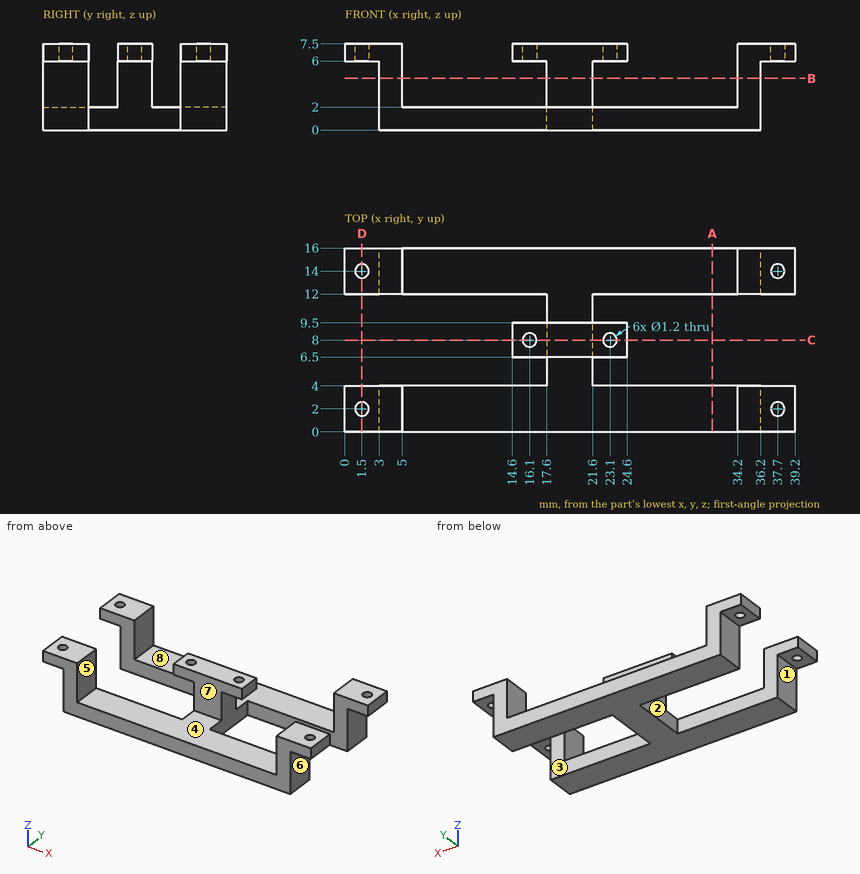
Input: dimensioned drawing with shaded views. Units: mm. Origin: part minimum x, y, z. A direction names the side the tool comes from. Give positions to 0.01 mm unless a question says otherwise; leave off trailing zeros. Order: outer loops, then holes, each group sorted by start corner. A loop starts at its lowest first (then second) coordinate and runs counter-clockwise, first axis right, second up. Notation, with made-up numbers: (28, -37) -> (40, -37) arc R12 cw to (40, -24) -> close; hole circle Ø3 at (65.5, -35.5). An arc over 180 degrees is marked (long way). Use a Markdown table: item, result.
1) Reachability of the marked faces 1, 2, 3, 4 and 5 from +Z, -Z, +X, -X, +Y, -Y: full face, straight path, thin tool, end or side. Return the list, or none.
Answer list:
| item | result |
|---|---|
| face 1 | -Z, -X, +Y, -Y |
| face 2 | -Z, -X |
| face 3 | +Z, -Z, +X |
| face 4 | +Z, -Y |
| face 5 | +Z, +Y, -Y |
2) Section query B-B, the plane z = 4.5. Return the cut outline in (x, y).
Answer list:
| item | result |
|---|---|
| outline | (3, 0) -> (5, 0) -> (5, 4) -> (3, 4) -> close; (3, 12) -> (5, 12) -> (5, 16) -> (3, 16) -> close; (17.6, 6.5) -> (21.6, 6.5) -> (21.6, 9.5) -> (17.6, 9.5) -> close; (34.2, 0) -> (36.2, 0) -> (36.2, 4) -> (34.2, 4) -> close; (34.2, 12) -> (36.2, 12) -> (36.2, 16) -> (34.2, 16) -> close |
3) Section query D-D, the plane x = 1.5. Return the cut outline in (y, z), then the cut area to 3 significant figures.
Answer list:
| item | result |
|---|---|
| outline | (0, 6) -> (1.4, 6) -> (1.4, 7.5) -> (0, 7.5) -> close; (2.6, 6) -> (4, 6) -> (4, 7.5) -> (2.6, 7.5) -> close; (12, 6) -> (13.4, 6) -> (13.4, 7.5) -> (12, 7.5) -> close; (14.6, 6) -> (16, 6) -> (16, 7.5) -> (14.6, 7.5) -> close |
| area | 8.40 mm² |
4) Section query A-A, the plane x = 32. Return the cut outline in (y, z).
Answer list:
| item | result |
|---|---|
| outline | (0, 0) -> (4, 0) -> (4, 2) -> (0, 2) -> close; (12, 0) -> (16, 0) -> (16, 2) -> (12, 2) -> close |
5) Contact query for flat-ended pins moving along their axis: P1, Ø4.5, axis at y = 3, z = 2.5, coming from the +X side; P2, Ø4, axis at x = 8.5, z = 6, coming from the -Y side; P3, Ø1.8, axis at y = 10, z = 3.5, coming from the +X side; P4, Ø3, axis at y = 1, z = 2.5, coming from the -X side. Output: stop coordinate, or through.
Answer list:
| item | result |
|---|---|
| P1 | x = 36.2 |
| P2 | through |
| P3 | x = 21.6 |
| P4 | x = 3 |
6) Section query C-C, the plane y = 8. Return the cut outline in (x, z).
Answer list:
| item | result |
|---|---|
| outline | (14.6, 6) -> (15.5, 6) -> (15.5, 7.5) -> (14.6, 7.5) -> close; (16.7, 6) -> (17.6, 6) -> (17.6, 0) -> (21.6, 0) -> (21.6, 6) -> (22.5, 6) -> (22.5, 7.5) -> (16.7, 7.5) -> close; (23.7, 6) -> (24.6, 6) -> (24.6, 7.5) -> (23.7, 7.5) -> close |
7) Mould query, pull axis X, two halves, no side actions, for the marked faces 6, 7 and 8. Classes: +X half, -X half, draft (parallel to the pull), parting line (faces both ways), or undercut.
Answer list:
| item | result |
|---|---|
| face 6 | +X half |
| face 7 | draft |
| face 8 | undercut |
8) Ray query, line 1 along Y through (x, z) = (37.7, 6.45); line 2 along Y through (x, z) = (14, 1.25); line 3 along X through (y, z) = (3.5, 5). Return the intervals inside material, ascending. Write a range as [from, to].
Answer list:
| item | result |
|---|---|
| line 1 | [0, 1.4], [2.6, 4], [12, 13.4], [14.6, 16] |
| line 2 | [0, 4], [12, 16] |
| line 3 | [3, 5], [34.2, 36.2] |
